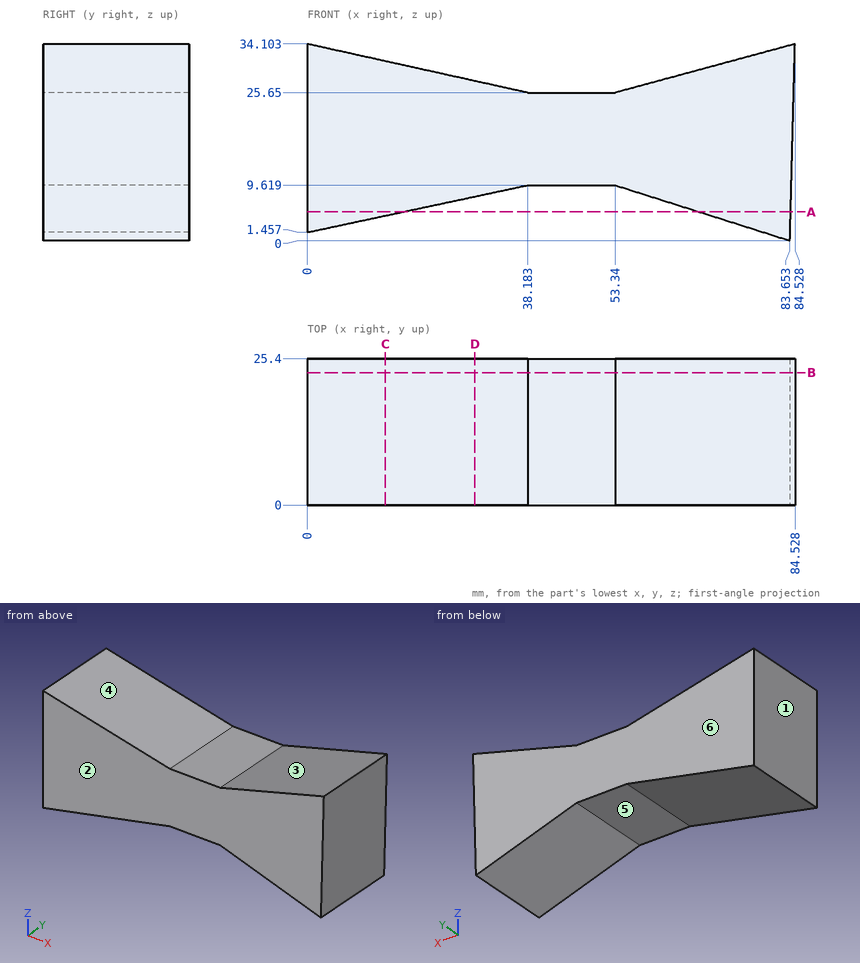
Source: three-view drawing plus pictorial views. Frame: mm from the lowest corner of the part. A direction names the side the tool comes from. Give positions to 0.01 mm unless a question says otherwise; leave off trailing zeros. Order: outer loops, then holes, each group sorted by start corner. A loop starts at its lowest first (then second) coordinate and runs counter-clockwise, first axis right, second up. Notation, with made-up numbers: M -10,-35 L 34,-35 A28 cw 34,-4 Z; hole C 21.5,-25.5 d7. An arc over 180 degrees is marked long. Return JSON: item names as keys, results as strings.
1) Section query C-C on x = 13.5. Output: boundary loops of the cut face in (y, z), and give its area (3 significant figures).
Taken from the geometry:
{"outline": "M 0,4.34 L 25.4,4.34 L 25.4,31.11 L 0,31.11 Z", "area": "680 mm2"}
2) Section query A-A on z = 5. Output: boundary loops of the cut face in (x, y) (1 decimal).
Taken from the geometry:
{"outline": "M 0,0 L 16.6,0 L 16.6,25.4 L 0,25.4 Z; M 67.9,0 L 83.8,0 L 83.8,25.4 L 67.9,25.4 Z"}
3) Section query B-B on y = 23. Output: boundary loops of the cut face in (x, z).
Taken from the geometry:
{"outline": "M 0,1.46 L 38.18,9.62 L 53.34,9.62 L 83.65,0 L 84.53,34.1 L 53.34,25.65 L 38.18,25.65 L 0,34.1 Z"}
4) Contact query for flat-ended pins moving along their axis: pin 1 (6 mm diameter, centred on x = 16.5, y = 22.5, fed in from -Z); pin 2 (1.5 mm diameter, centred on x = 21.5, y = 5, fed in from +Z); pin 3 (10 mm diameter, centred on x = 21, y = 16.5, fed in from -Z). Output: stop coordinate, or through.
Taken from the geometry:
{"pin 1": "stops at z = 4.34", "pin 2": "stops at z = 29.51", "pin 3": "stops at z = 4.88"}
5) Mould query, pull axis X, two halves, no side actions, for the marked faces 1, 2 and 3. Classes: released by +X, released by -X, zero draft, split by the parting line, or undercut.
Taken from the geometry:
{"face 1": "released by -X", "face 2": "zero draft", "face 3": "undercut"}
6) Section query D-D on x = 29. Output: boundary loops of the cut face in (y, z) (1 decimal), and give its area (3 significant figures).
Taken from the geometry:
{"outline": "M 0,7.7 L 25.4,7.7 L 25.4,27.7 L 0,27.7 Z", "area": "509 mm2"}
7) Line query: L1, parallel to Z at x = 48.5, y = 10.75; L2, parallel to Z at x = 26, y = 13.75 (1 decimal); L3, parallel to X at y = 11.5, z = 16. Output: solid intervals per line, ascending. Write a range as [from, to].
Taken from the geometry:
{"L1": "z = [9.62, 25.65]", "L2": "z = [7, 28.3]", "L3": "x = [0, 84.06]"}
8) Access query for the marked faces 4, 5 and 6. Directions: +Z, -Z, +X, -X, +Y, -Y. A direction counts if a zero-diameter tool reaches every point of the face in a straight line with its end or side. Return the directions, or none.
Taken from the geometry:
{"face 4": "+Z, +Y, -Y", "face 5": "-Z, +Y, -Y", "face 6": "+Z, -Z, +X, -X, +Y"}
